CAD build for the part. Positions are in the model's coordinates, mm. A direction names the side the tool comes from. Round coordinates to 2 decimals unless told otherwise and drop trailing zeros. Write each loop counter-clockwise with the first axis right and the second up, starting at its lowest first coordinate (ties: lowest second). Pieces come first, ordered by that corner, then holes. Notation, with made-up numbers: (35, -6.75) - (79, -6.75) arc R17 ccw to (79, 6.25) - close; hole circle Ø6 at (-35, -26). An arc over 180 degrees is marked (long way). Put each result on its own line as item: value. Start each with the question number.
Item 1: Cut at D-D (x = 40). Give the cut face in (y, z).
Item 2: Mould opens along X. For faces 4 (the flat face through (33.726, 21, 1)), 5 (the cylindrical face through (26.578, 38.771, 1.479)), 6 (the flat face through (29, -35.522, 1)), 7 (the flat face through (56.026, -2, 1)) say: released by +X, released by -X, zero draft, split by the parting line, or undercut.
Item 3: Cut at A-A (y = 22.5). Give the cut face in (x, z).
Item 4: Cut at B-B (x = 36). Give the cut face in (y, z).
Item 5: 3-axis set-ups, long thin cutter, end or side, ignore diameter. For faces 1 (the flat face through (40, 41.778, 1)), 2 (the flat face through (40, 32.078, 1)), 3 (the flat face through (34.876, -34, 1)): which of +Z, -Z, +X, -X, +Y, -Y reach the whole face in a straight line?
Item 6: Drill centre lines: line 1 (X direction, y = 23, z = 0.75); line 2 (Y direction, x = 39, z = 2.6); line 3 (Y direction, x = 36, z = 2.1). Where is each one in solid material? Low to high. Write a range as from..to.
Item 7: Cut at C-C (z = 2.4). Give the cut face in (x, y).
Autodesk Inventor part; units mm, degrees
ref_plane "YZ Plane" through (0, 0, 0) normal (1, 0, 0) x (0, 1, 0)
ref_plane "XZ Plane" through (0, 0, 0) normal (0, 1, 0) x (-1, 0, 0)
ref_plane "XY Plane" through (0, 0, 0) normal (0, 0, 1) x (1, 0, 0)
sketch "Sketch1" plane through (0, 0, 0) normal (0, 0, 1) x (1, 0, 0)
  line L0 (46.0264, 41.778) -> (33.7264, 41.778)
  line L1 (23.7264, 31.778) -> (23.7264, -35.522)
  line L2 (56.0264, -35.522) -> (56.0264, 31.778)
  line L3 (46.0264, 32.078) -> (33.7264, 32.078)
  line L4 (33.7264, 32.078) -> (33.7264, 9.478)
  line L5 (33.7264, 9.478) -> (46.0264, 9.478)
  line L6 (46.0264, 9.478) -> (46.0264, 32.078)
  line L7 (46.0264, 32.078) -> (33.7264, 32.078) construction
  line L8 (33.7264, 32.078) -> (33.7264, 36.778) construction
  line L9 (33.7264, 36.778) -> (46.0264, 36.778) construction
  line L10 (46.0264, 36.778) -> (46.0264, 32.078) construction
  line L11 (39.8764, 36.778) -> (39.8764, 32.078) construction
  circle A0 centre (39.8764, 35.678) radius 1.1
  line L12 (46.0264, 9.478) -> (33.7264, 9.478) construction
  line L13 (33.7264, 9.478) -> (33.7264, 4.778) construction
  line L14 (33.7264, 4.778) -> (46.0264, 4.778) construction
  line L15 (46.0264, 4.778) -> (46.0264, 9.478) construction
  line L16 (39.8764, 4.778) -> (39.8764, 9.478) construction
  circle A1 centre (39.8764, 5.878) radius 1.1
  arc A2 (33.7264, 41.778) -> (23.7264, 31.778) centre (33.7264, 31.778) ccw
  arc A3 (56.0264, 31.778) -> (46.0264, 41.778) centre (46.0264, 31.778) ccw
  line L17 (34.8764, -35.522) -> (34.8764, -32.522)
  line L18 (34.8764, -32.522) -> (44.8764, -32.522)
  line L19 (44.8764, -32.522) -> (44.8764, -35.522)
  line L20 (23.7264, -35.522) -> (34.8764, -35.522)
  line L21 (44.8764, -35.522) -> (56.0264, -35.522)
  point P0 (0, 0)
  dimension "d0" = 12.3
  dimension "d1" = 22.6
  dimension "d2" = 4.7
  dimension "d3" = 1.1
  dimension "d4" = 4.7
  dimension "d5" = 1.1
  dimension "d7" = 5
  dimension "d8" = 10
  dimension "d9" = 10
  dimension "d10" = 10
  dimension "d11" = 32.3
  dimension "d12" = 10
  dimension "d13" = 11.15
  dimension "d14" = 11.15
  dimension "d17" = 45
  dimension "d18" = 45
  dimension "d20" = 42
  dimension "d21" = 12.3
  dimension "d22" = 12.3
extrude "Extrusion1" add sketch "Sketch1" along normal blind 3
properties part number "Stutze_Servo"
Output values:
1. outline: (-32.52, 0) - (4.78, 0) - (4.78, 3) - (-32.52, 3) - close; (6.97, 0) - (9.48, 0) - (9.48, 3) - (6.97, 3) - close; (32.08, 0) - (34.58, 0) - (34.58, 3) - (32.08, 3) - close; (36.77, 0) - (41.78, 0) - (41.78, 3) - (36.77, 3) - close
2. face 4: undercut
2. face 5: released by -X
2. face 6: zero draft
2. face 7: released by +X
3. outline: (23.73, 0) - (33.73, 0) - (33.73, 3) - (23.73, 3) - close; (46.03, 0) - (56.03, 0) - (56.03, 3) - (46.03, 3) - close
4. outline: (-32.52, 0) - (9.48, 0) - (9.48, 3) - (-32.52, 3) - close; (32.08, 0) - (41.78, 0) - (41.78, 3) - (32.08, 3) - close
5. face 1: +Z, -Z, +X, -X, +Y
5. face 2: +Z, -Z
5. face 3: +Z, -Z, -Y
6. line 1: 23.73..33.73, 46.03..56.03
6. line 2: -32.52..5.21, 6.54..9.48, 32.08..35.01, 36.34..41.78
6. line 3: -32.52..9.48, 32.08..41.78
7. outline: (23.73, -35.52) - (34.88, -35.52) - (34.88, -32.52) - (44.88, -32.52) - (44.88, -35.52) - (56.03, -35.52) - (56.03, 31.78) arc R10 ccw to (46.03, 41.78) - (33.73, 41.78) arc R10 ccw to (23.73, 31.78) - close; hole (33.73, 9.48) - (46.03, 9.48) - (46.03, 32.08) - (33.73, 32.08) - close; hole circle Ø2.2 at (39.88, 5.88); hole circle Ø2.2 at (39.88, 35.68)
